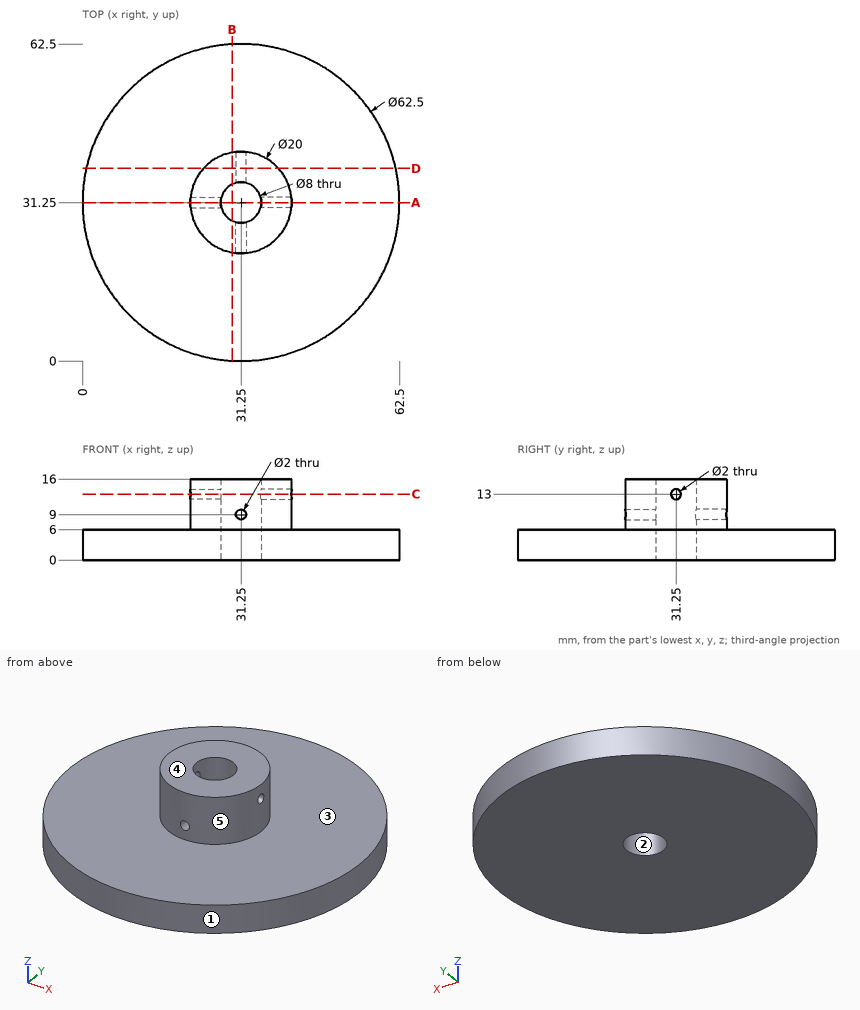
Geometry check sheet. Reference: drawing and pictorial views, mm from the part's lowest x, y, z. A direction names the side the tool comes from. Give positions to 0.01 mm unless a question says otherwise; leave off trailing zeros. Write each loop counter-clockwise with the first axis right and the second up, starting at its lowest first coordinate (ties: lowest second). Pieces come first, ordered by that corner, then holes. Notation, with made-up numbers: M -38,57 L -34,57 A23 cw -34,89 Z; hole C -30.75,-37 d7. An arc over 180 degrees is marked long. Answer as CSV lines item,"result". Start each with the question number.
Q1. Material ranges on L1, parallel to Z at x = 6, y = 24.5; L2, parallel to Z at x = 31.25, y = 25.5; L3, parallel to Y at x = 31.25, z = 3.5, recorded low to high.
Q2. Section check B-B, the plane x = 29.5. Record the cut outline in (y, z), then the cut area to 3 significant figures.
Q3. Go/stop test with flat-tipped pins: pin 1 (3 mm diameter, centred on y = 31.25, z = 13, fed in from +X); pin 2 (4 mm diameter, centred on x = 22, z = 7.5, fed in from +Y); pin 3 (5 mm diameter, centred on y = 8, z = 5, fed in from +X). Record where each tip stops, or that it passes through.
Q4. Tool access check on the marked faces 4 and 5. Record the directions out of +Z, -Z, +X, -X, +Y, -Y that give a thin tool (end or side, any length) a straight path to the whole face; none if there is none.
Q5. Release check for a two-part mould opening along X. For the marked faces 1, 2 and 3 record: pulls with the +X half, pulls with the -X half, needs draft (parallel to the pull), parting line crosses it, or undercut.
Q6. Section check D-D, the plane y = 38. Record the cut outline in (x, z).
Q7. Section check C-C, the plane z = 13. Record the cut outline in (x, y), then the cut area to 3 significant figures.
Q8. Section check A-A, the plane y = 31.25. Record the cut outline in (x, z), then the cut area to 3 significant figures.
Geometry says:
1,L1,"0 to 6"
1,L2,"0 to 8, 10 to 16"
1,L3,"0 to 27.25, 35.25 to 62.5"
2,outline,"M 0.05,0 L 27.65,0 L 27.65,16 L 21.4,16 L 21.4,6 L 0.05,6 Z; M 34.85,0 L 62.45,0 L 62.45,6 L 41.1,6 L 41.1,16 L 34.85,16 Z"
2,area,"456 mm^2"
3,pin 1,"x = 41.25"
3,pin 2,"y = 61.48"
3,pin 3,"x = 54.62"
4,face 4,"+Z, +X, -X, +Y, -Y"
4,face 5,"+Z"
5,face 1,"parting line crosses it"
5,face 2,"undercut"
5,face 3,"needs draft"
6,outline,"M 0.74,0 L 61.76,0 L 61.76,6 L 38.63,6 L 38.63,16 L 23.87,16 L 23.87,6 L 0.74,6 Z; hole C 31.25,9 d2"
7,outline,"M 21.3,30.25 A10 ccw 41.2,30.25 L 35.12,30.25 A4 cw 27.38,30.25 Z; M 21.3,32.25 L 27.38,32.25 A4 cw 35.12,32.25 L 41.2,32.25 A10 ccw Z"
7,area,"240 mm^2"
8,outline,"M 0,0 L 27.25,0 L 27.25,12 L 21.25,12 L 21.25,6 L 0,6 Z; M 21.25,14 L 27.25,14 L 27.25,16 L 21.25,16 Z; M 35.25,0 L 62.5,0 L 62.5,6 L 41.25,6 L 41.25,12 L 35.25,12 Z; M 35.25,14 L 41.25,14 L 41.25,16 L 35.25,16 Z"
8,area,"423 mm^2"
